Autodesk Inventor part; units mm, degrees
ref_plane "YZ Plane" through (0, 0, 0) normal (1, 0, 0) x (0, 1, 0)
ref_plane "XZ Plane" through (0, 0, 0) normal (0, 1, 0) x (-1, 0, 0)
ref_plane "XY Plane" through (0, 0, 0) normal (0, 0, 1) x (1, 0, 0)
sketch "Sketch1" plane through (0, 0, 0) normal (0, 0, 1) x (1, 0, 0)
  line L0 (-45, 35) -> (69, 35)
  line L1 (69, 35) -> (69, -18)
  line L2 (65, -22) -> (-41, -22)
  line L3 (-45, -18) -> (-45, 35)
  arc A0 (-45, -18) -> (-41, -22) centre (-41, -18) ccw
  arc A1 (65, -22) -> (69, -18) centre (65, -18) ccw
  point P0 (0, 0)
  dimension "d0" = 114
  dimension "d1" = 4
  dimension "d2" = 4
  dimension "d3" = 57
extrude "Plate1" add sketch "Sketch1" along normal blind 4
sketch "Sketch2" plane through (0, 0, 4) normal (0, 0, 1) x (1, 0, 0)
  line L0 (69, 35) -> (-45, 35)
  arc A0 (-7, 35) -> (31, 35) centre (12, 35) ccw
  point P0 (0, 0)
  dimension "d5" = 38
extrude "Extrusion1" cut sketch "Sketch2" against normal through all
equation "\"d4\" = Thickness"
equation "\"BendRadius\" = Thickness"
equation "\"BendReliefWidth\" = Thickness"
equation "\"BendReliefDepth\" = 0.5 * Thickness"
equation "\"CornerReliefSize\" = 4 * Thickness"
equation "\"MinimumRemnant\" = 2 * Thickness"
equation "\"TransitionRadius\" = BendRadius"
equation "\"JacobiRadiusSize\" = BendRadius"
equation "\"GapSize\" = Thickness"
properties part number "Bottom joint housing cover_ final"
Here's how the part is built. I have some questions about the finished solid (model axes, mm). Give positions to 0.01 mm unless a question says otherwise; leave off trailing zeros. Order: outer loops, then holes, each group sorted by start corner. A loop starts at its lowest first (then second) coordinate and runs counter-clockwise, first axis right, second up. Notation, with made-up numbers: (-34, -30) -> (-20, -30) arc R20 ccw to (-20, 4) -> close; hole circle Ø2 at (59, 36.5). An arc over 180 degrees is marked (long way). Use CSV: the item, a comma, the result in double quotes. Start each with the question number.
Item 1: I'm going to push a flat-ended pin straight in: P1, Ø1.5, axis at x = 38.5, y = 20.5, coming from the -Z side. Where does the tip first touch, or does it pass through?
Item 2: Suppose I cut it at B-B (y = 21). List the corners of the cut face in (x, z) for me, and give its area (3 significant figures).
Item 3: If I drill on probe 1 along X at (y, z) = (32, 3.6); probe 2 along X at (y, z) = (22, 2.2); probe 3 along Y at (x, z) = (22, 1.45), over which ranges is the centre line in solid material (lowest first)? Write a range as [from, to].
Item 4: Suppose I cut it at A-A (z = 1.45). List the corners of the cut face in (x, y) for me, and give its area (3 significant figures).
Item 5: Suppose I cut it at C-C (x = 12). List the corners of the cut face in (y, z) for me, and give its area (3 significant figures).
Item 6: Thinking about a two-plate mould opening in X: for faces 1 (the flat face through (-45, 8, 2)), 2 (the flat face through (-26, 35, 2)), 3 (the cylindrical face through (12, 16, 2)), 4 (the flat face through (69, 9, 2)), which applies, pulls with the +X half, pulls with the -X half, needs draft (parallel to the pull), parting line crosses it, or undercut?
Answer block:
1,P1,"stops at z = 0"
2,outline,"(-45, 0) -> (-0.85, 0) -> (-0.85, 4) -> (-45, 4) -> close; (24.85, 0) -> (69, 0) -> (69, 4) -> (24.85, 4) -> close"
2,area,"353 mm^2"
3,probe 1,"x = [-45, -6.76], [30.76, 69]"
3,probe 2,"x = [-45, -1.86], [25.86, 69]"
3,probe 3,"y = [-22, 18.84]"
4,outline,"(-45, -18) arc R4 ccw to (-41, -22) -> (65, -22) arc R4 ccw to (69, -18) -> (69, 35) -> (31, 35) arc R19 cw to (-7, 35) -> (-45, 35) -> close"
4,area,"5,920 mm^2"
5,outline,"(-22, 0) -> (16, 0) -> (16, 4) -> (-22, 4) -> close"
5,area,"152 mm^2"
6,face 1,"pulls with the -X half"
6,face 2,"needs draft"
6,face 3,"undercut"
6,face 4,"pulls with the +X half"
